Answer from the drawing. Dimensions are ordinates in mm from the lowest x, y and z of the part. Coordinates: 2 decimals unless noted, no trailing zeros. Write each loop counter-clockwise with the first axis right and the second up, starting at its lowest first coordinate (ties: lowest second). Pieces come first, ordered by that corner, then holes.
(1) The part is cut by section A-A on x = 49. Determine the outline of the cut face in (y, z), plus the area to 3 significant figures.
(2) Straight lines are drawn through the part: line 1 (Y direction, x = 43, z = 495); line 2 (X direction, y = 81, z = 844.5). For each, find the intervals that lie inside material, in ascending order.
(3) The part is cut by section B-B on z = 826. Determine the outline of the cut face in (x, y).
(4) Given P1, Ø4, axis at y = 76.5, z = 217, coming from the +X side; P2, Ø8, axis at y = 99.5, z = 891, coming from the -X side, each flat-ended and moving along its own axis, determine where each tip first touches the part or whether it passes through.
(5) The part is cut by section C-C on y = 84.5. Determine the outline of the cut face in (x, z).
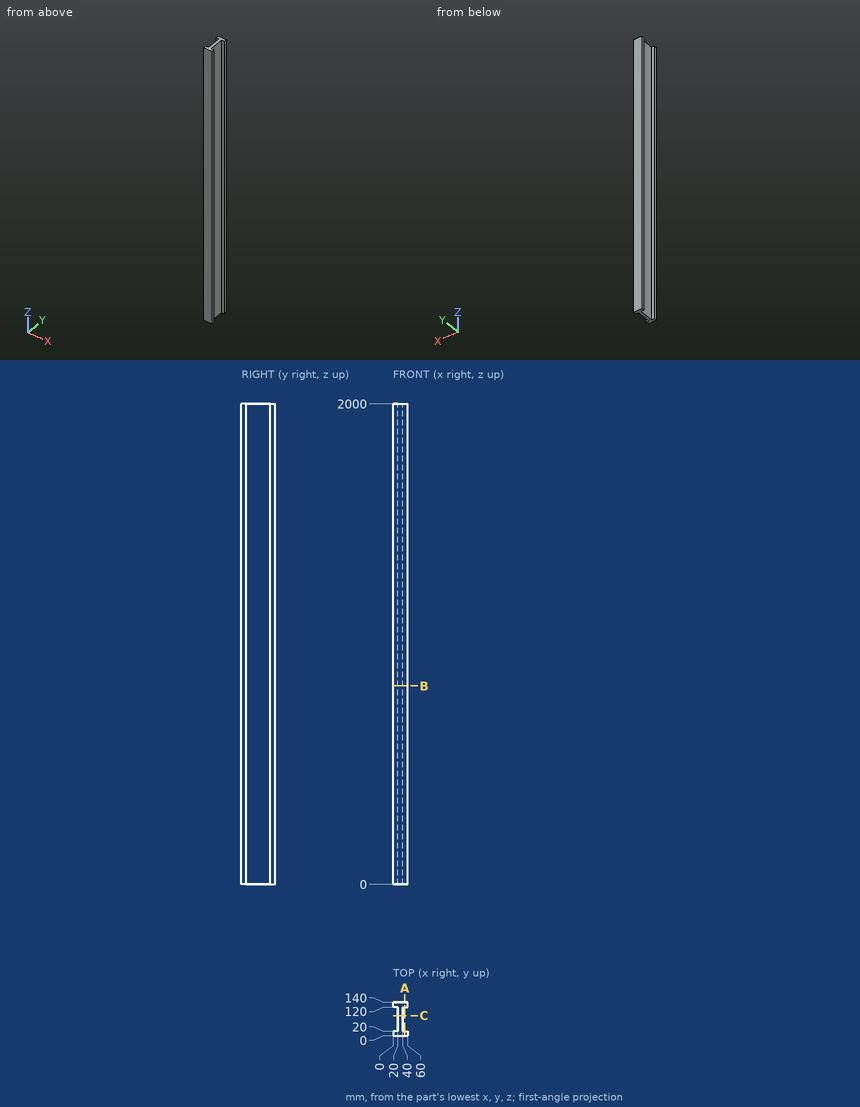
Model answer:
1. outline: (0, 0) - (20, 0) - (20, 2000) - (0, 2000) - close; (120, 0) - (140, 0) - (140, 2000) - (120, 2000) - close
1. area: 80,000 mm2
2. line 1: y = 0 to 20, 120 to 140
2. line 2: x = 20 to 40
3. outline: (0, 0) - (60, 0) - (60, 20) - (40, 20) - (40, 120) - (60, 120) - (60, 140) - (0, 140) - (0, 120) - (20, 120) - (20, 20) - (0, 20) - close
4. P1: stops at x = 40
4. P2: stops at x = 20
5. outline: (20, 0) - (40, 0) - (40, 2000) - (20, 2000) - close
